```python
from build123d import *

# Parameters (mm, degrees)
SKETCH1_R               = 1.45
BOSS_EXTRUDE1_DEPTH     = 7
SKETCH3_R               = 2.065
BOSS_EXTRUDE3_DEPTH     = 8
FILLET1_SIZE            = 3
FILLET1_SIZE_2          = 1
CUT_EXTRUDE1_DEPTH      = 1.5
CUT_EXTRUDE1_DEPTH_BACK = 1.5
SKETCH5_R               = 1.280712692
FILLET2_R               = 0.25


with BuildPart() as part:
    # Sketch1 → Boss-Extrude1 (new body)
    with BuildSketch(Plane(origin=(0, 0, 0), x_dir=(1, 0, 0), z_dir=(0, 1, 0))):
        with Locations(Location((0, 0, 0), (0, 0, 270))):
            Circle(SKETCH1_R)
    extrude(amount=BOSS_EXTRUDE1_DEPTH)

    # Sketch3 → Boss-Extrude3 (add)
    with BuildSketch(Plane(origin=(0, 7, 0), x_dir=(1, 0, 0), z_dir=(0, 1, 0))):
        with Locations(Location((0, 0, 0), (0, 0, 270))):
            Circle(SKETCH3_R)
    extrude(amount=BOSS_EXTRUDE3_DEPTH)

    # Fillet1
    # an asymmetric fillet: 3, 1 mm, written as the material it takes off along each edge
    with BuildSketch(Plane(origin=(0, 0, 0), x_dir=(0, 0, 1), z_dir=(-1, 0, 0))) as fillet1_piece_1:
        with BuildLine():
            Bezier((1.45, FILLET1_SIZE), (1.45, 0), (1.45 - FILLET1_SIZE_2, 0), weights=[1, 0.707106781, 1])
            Line((1.45 - FILLET1_SIZE_2, 0), (1.45, 0))
            Line((1.45, 0), (1.45, FILLET1_SIZE))
        make_face()
    revolve(axis=Axis((0, 0, 0), (0, 1, 0)), mode=Mode.SUBTRACT)

    # Sketch5 → Cut-Extrude1 (cut, two sides: drawn at the far end of the back side and taken through both)
    with BuildSketch(Plane(origin=(0, 0, 0), x_dir=(0, 0, -1), z_dir=(1, 0, 0)).offset(-CUT_EXTRUDE1_DEPTH_BACK)):
        with Locations((0, 15.2)):
            Circle(SKETCH5_R)
    extrude(amount=CUT_EXTRUDE1_DEPTH + CUT_EXTRUDE1_DEPTH_BACK, mode=Mode.SUBTRACT)

    # Fillet2
    # the kernel refuses this fillet: 0.25 mm, written as the material it takes off along each edge
    with BuildSketch(Plane(origin=(1.5, 15, 1.265), x_dir=(0, 0, 1), z_dir=(-1, 0, 0)), Plane(origin=(-1.5, 15, -1.265), x_dir=(0, 0, -1), z_dir=(1, 0, 0))) as fillet2_piece_1:
        with BuildLine():
            CenterArc((0.19807257, -0.25), FILLET2_R, 90, 72.903573808)
            Line((-0.040880268, -0.176504823), (-0.045659325, -0.17503492))
            ThreePointArc((-0.045659325, -0.17503492), (-0.022186102, -0.087848028), (-0.004938656, 0.000780815))
            Line((-0.004938656, 0.000780815), (0, 0.005))
            Line((0, 0.005), (0.19807257, 0.005))
            Line((0.19807257, 0.005), (0.19807257, 0))
        make_face()
    extrude(amount=3, mode=Mode.SUBTRACT)


solid = part.part
```
Geometry check sheet. Reference: the model listing, model coordinates, mm. A direction names the side the tool comes from. Coordinates: 2 decimals unless noted, no trailing zeros. Write each loop counter-clockwise with the first axis right and the second up, starting at its lowest first coordinate (ties: lowest second). Pieces come first, ordered by that corner, then holes. Notation, with made-up numbers: M 53,-4 L 96,-4 A28 cw 96,26 Z; hole C 81.25,-27 d5. An arc over 180 degrees is marked long. One line per item, written item: value. Start each with the question number.
(1) Depth check by flat-ended pin: pin 1 (1 mm diameter, centred on x = -0.5, z = 0.5, fed in from +Y). Enter the tip coordinate at first touch or a pass-through.
(2) Sectioned sample at D-D, the plane y = 5.75. Enter the section's corners in (x, z), and give its area (3 significant figures).
(3) Tool access check on faces 1 (the face through (1.5, 14.6, 0)), 2 (the face through (-1.257, 10.944, -1.639)). Record the directions out of +Z, -Z, +X, -X, +Y, -Y that give a thin tool (end or side, any length) a straight path to the whole face; none if there is none.
(4) Release check for a two-part mould opening along X. For faces 3 (the face through (-1.35, 7, 0.89)), 4 (the face through (0.06, 4.97, -1.45)), 5 (the face through (-1.5, 14.6, 0)) record: released by +X, released by -X, zero draft, split by the parting line, or undercut.
(5) Scan lines: line 1 along X through (y, z) = (6.5, 0.3); line 2 along Y through (x, z) = (0.2, 1.8). Record each from-to range of solid material in increasing order. Write a range as [from, to].
(6) Sectioned sample at C-C, the plane z = -1.65. Enter the section's corners in (x, y), and give its area (3 significant figures).
(7) Sectioned sample at B-B, the plane x = -1.8. Enter the section's corners in (y, z), and give its area (3 significant figures).
(8) Sectioned sample at A-A, the plane y = 8. Enter the section's corners in (x, z) (3 decimals), and give its area (3 significant figures).
Filled sheet:
1. pin 1: y = 14.4
2. outline: C 0,0 d2.9
2. area: 6.61 mm²
3. face 1: +Y
3. face 2: +Y, -Y
4. face 3: zero draft
4. face 4: split by the parting line
4. face 5: undercut
5. line 1: [-1.42, 1.42]
5. line 2: [7, 15]
6. outline: M -1.24,7 L 1.24,7 L 1.24,15 L -1.24,15 Z
6. area: 19.9 mm²
7. outline: M 7,-1.01 L 15,-1.01 L 15,1.01 L 7,1.01 Z
7. area: 16.2 mm²
8. outline: C 0,0 d4.13
8. area: 13.4 mm²
